```python
from build123d import *

# Parameters (mm, degrees)
SKETCH1_R               = 24
SKETCH1_R_2             = 22
BOSS_EXTRUDE1_DEPTH     = 161
CUT_EXTRUDE1_DEPTH      = 161
CUT_EXTRUDE1_DEPTH_BACK = 161
CUT_EXTRUDE2_DEPTH      = 161
CUT_EXTRUDE3_DEPTH      = 161
CUT_EXTRUDE3_DEPTH_BACK = 161


with BuildPart() as part:
    # Sketch1 → Boss-Extrude1 (new body)
    with BuildSketch(Plane.XY):
        with BuildLine():
            Line((-179.511953074, -16.515594264), (185.913473281, -26.726946149))
            ThreePointArc((185.913473281, -26.726946149), (248.5, 0), (185.913473281, 26.726946149))
            Line((185.913473281, 26.726946149), (-179.511953074, 16.515594264))
            ThreePointArc((-179.511953074, 16.515594264), (-247.5, 0), (-179.511953074, -16.515594264))
        make_face()
        with Locations((-211.5, 0)):
            Circle(SKETCH1_R, mode=Mode.SUBTRACT)
        with Locations((211.5, 0)):
            Circle(SKETCH1_R_2, mode=Mode.SUBTRACT)
    extrude(amount=-BOSS_EXTRUDE1_DEPTH)

    # Sketch3 → Cut-Extrude1 (cut, two sides: drawn at the far end of the back side and taken through both)
    with BuildSketch(Plane(origin=(-0.601210303, 21.515028947, 0), x_dir=(0.9996098022907813, 0.027932833085548846, 0), z_dir=(-0.027932833085548846, 0.9996098022907813, 0)).offset(-CUT_EXTRUDE1_DEPTH_BACK)):
        Polygon((-178.980580584, 135.5), (-268.840136548, 135.5), (-268.840136548, 212.571288089), (186.587489595, 212.571288089), (186.587489595, 161), align=None)
        Polygon((-178.980580584, 25.5), (-268.840136548, 25.5), (-268.840136548, -47.637415265), (186.587489595, -47.637415265), (186.587489595, 0), align=None)
    extrude(amount=CUT_EXTRUDE1_DEPTH + CUT_EXTRUDE1_DEPTH_BACK, mode=Mode.SUBTRACT)

    # Sketch4 → Cut-Extrude2 (cut)
    with BuildSketch(Plane(origin=(-0.601210303, 21.515028947, 0), x_dir=(0.9996098022907813, 0.027932833085548846, 0), z_dir=(-0.027932833085548846, 0.9996098022907813, 0))):
        with BuildLine():
            Line((-121.980580584, 65.23825231), (-121.980580584, 95.76174769))
            ThreePointArc((-121.980580584, 95.76174769), (-116.606484769, 109.402969291), (-103.372287906, 115.713267701))
            Line((-103.372287906, 115.713267701), (125.195782273, 131.656907928))
            ThreePointArc((125.195782273, 131.656907928), (140.228711197, 126.331292103), (146.587489595, 111.705387918))
            Line((146.587489595, 111.705387918), (146.587489595, 48.31804977))
            ThreePointArc((146.587489595, 48.31804977), (140.197596355, 33.6631873), (125.110990195, 28.372625495))
            Line((125.110990195, 28.372625495), (-103.457079984, 45.292828035))
            ThreePointArc((-103.457079984, 45.292828035), (-116.635443053, 51.628145551), (-121.980580584, 65.23825231))
        make_face()
    extrude(amount=-CUT_EXTRUDE2_DEPTH, mode=Mode.SUBTRACT)

    # Sketch6 → Cut-Extrude3 (cut, two sides: drawn at the far end of the back side and taken through both)
    with BuildSketch(Plane(origin=(-0.601210303, 21.515028947, 0), x_dir=(0.9996098022907813, 0.027932833085548846, 0), z_dir=(-0.027932833085548846, 0.9996098022907813, 0)).offset(-CUT_EXTRUDE3_DEPTH_BACK)):
        Polygon((172.587489595, 80.011718844), (172.587489595, 133.988681084), (279.945964302, 133.988681084), (279.945964302, 27.005225925), (172.587489595, 27.005225925), align=None)
    extrude(amount=CUT_EXTRUDE3_DEPTH + CUT_EXTRUDE3_DEPTH_BACK, mode=Mode.SUBTRACT)


solid = part.part
```
Geometry: final body of the model. Coordinates: model frame, mm. A direction names the side the tool comes from. Round coordinates to 2 decimals unless told otherwise and drop trailing zeros. Order: outer loops, then holes, each group sorted by start corner. A loop starts at its lowest first (then second) coordinate and runs counter-clockwise, first axis right, second up. Notation, with made-up numbers: (84.25, 74.5) -> (91.25, 74.5) arc R27 ccw to (91.25, 99.5) -> close; hole circle Ø8 at (-7.75, -3). An arc over 180 degrees is marked (long way). Use one line per item in the form item = value. Start each with the question number.
1. Line query: probe 1 along Y at (x, z) = (211.5, -19.5); probe 2 along X at (y, z) = (0.5, -55); probe 3 along X at (y, z) = (-19.5, -117). Output: solid intervals per line, ascending.
2. Pin query (flat end, axial travel): pin 1 Ø1.5 at (y, z) = (-0.5, -84) entering from +X; pin 2 Ø2 at (y, z) = (-9.5, -70.5) entering from +X; pin 3 Ø3 at (y, z) = (15, -114) entering from +X; pin 4 Ø2 at (x, y) = (-31, -22) entering from -Z. Return the tip coordinate at first contact, or that it passes through.
3. Draft query along Y for faces 4 (the face through (189.52, 0.97, -13.31)), 5 (the face through (248.48, -1.21, -147.31)), 6 (the face through (-235.477, 1.055, -79.73)), 7 (the face through (231, -16, -161)). Return one class per face: pulls with the +Y half, pulls with the -Y half, needs draft (parallel to the pull), parting line crosses it, or undercut.
4. Reachability of faces 1 (the face through (231, -16, 0)), 2 (the face through (-236, -1, -25.5)), 3 (the face through (-116.534, -0.118, -51.475)) from +Z, -Z, +X, -X, +Y, -Y: full face, straight path, thin tool, end or side. Return the list, or none.
5. Cut plane C-C (y = 0). Count the separate pieces of the cut face and the enclosed holes in it, then the cut area to 3 significant figures.
6. Cut plane A-A (x = 211.5). Return the cut outline in (y, z), then the cut area to 3 significant figures.
7. Cut plane D-D (z = -12.5). Return the cut outline in (x, y), then the cut area to 3 significant figures.
8. Cut plane B-B (x = -211.5). Return the cut outline in (y, z), then the cut area to 3 significant figures.
Solution:
q1.probe_1 = -37 to -22, 22 to 37
q1.probe_2 = -247.5 to -235.49, -187.51 to -119.22, 146.63 to 172.64
q1.probe_3 = -241.76 to -225.49, -197.51 to -181.24, 146.48 to 173.2
q2.pin_1 = 172.69
q2.pin_2 = 172.95
q2.pin_3 = 172.28
q2.pin_4 = through
q3.face_4 = undercut
q3.face_5 = parting line crosses it
q3.face_6 = undercut
q3.face_7 = needs draft
q4.face_1 = +Z, +X, -X, +Y, -Y
q4.face_2 = +Z, -X, +Y, -Y
q4.face_3 = +Y
q5.separate_pieces = 4
q5.enclosed_holes = 1
q5.area = 28,200 mm^2
q6.outline = (-37, -161) -> (-22, -161) -> (-22, -133.99) -> (-37, -133.99) -> close; (-37, -27.01) -> (-22, -27.01) -> (-22, 0) -> (-37, 0) -> close; (22, -161) -> (37, -161) -> (37, -133.99) -> (22, -133.99) -> close; (22, -27.01) -> (37, -27.01) -> (37, 0) -> (22, 0) -> close
q6.area = 1,620 mm^2
q7.outline = (6.78, 21.72) -> (8, -21.76) -> (185.91, -26.73) arc R37 ccw (long way) to (185.91, 26.73) -> close; hole circle Ø44 at (211.5, 0)
q7.area = 11,000 mm^2
q8.outline = (-36, -135.5) -> (-24, -135.5) -> (-24, -25.5) -> (-36, -25.5) -> close; (24, -135.5) -> (36, -135.5) -> (36, -25.5) -> (24, -25.5) -> close
q8.area = 2,640 mm^2
